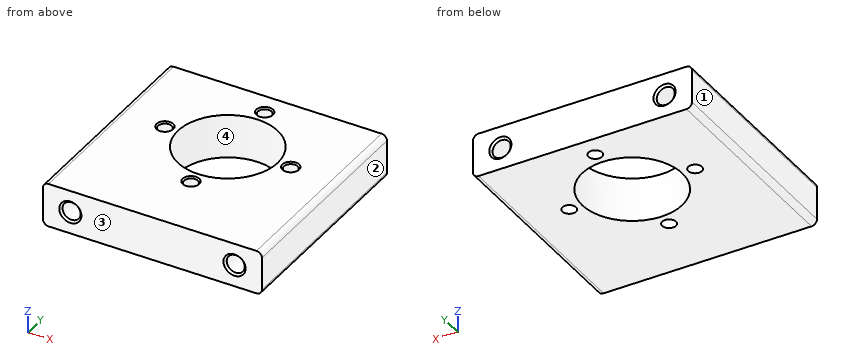
from build123d import *

# Parameters (mm, degrees)
SKETCH_1_W                   = 40
SKETCH_1_H                   = 8
EXTRUDE_1_DEPTH              = 39
HOLE_WIZARD_M4_1_D           = 3.3
HOLE_WIZARD_M4_1_DEPTH       = 9.108579979
HOLE_WIZARD_M4_1_CSINK_D     = 4.05
HOLE_WIZARD_M4_1_CSINK_ANGLE = 90
HOLE_WIZARD_M4_1_TIP         = 0.991420021
SKETCH_5_R                   = 9.125
CUT_EXTRUDE_1_DEPTH          = 39
HOLE_WIZARD_M4_2_D           = 3.3
HOLE_WIZARD_M4_2_DEPTH       = 9.108579979
HOLE_WIZARD_M4_2_CSINK_D     = 4.05
HOLE_WIZARD_M4_2_CSINK_ANGLE = 90
HOLE_WIZARD_M4_2_TIP         = 0.991420021
HOLE_WIZARD_M3_1_D           = 2.5
HOLE_WIZARD_M3_1_CSINK_D     = 3.05
HOLE_WIZARD_M3_1_CSINK_ANGLE = 90
FILLET_1_R                   = 1


with BuildPart() as part:
    # 草图1 → 凸台-拉伸1 (new body)
    with BuildSketch(Plane(origin=(0, 0, 0), x_dir=(1, 0, 0), z_dir=(0, 1, 0))):
        Rectangle(SKETCH_1_W, SKETCH_1_H)
    extrude(amount=EXTRUDE_1_DEPTH)

    # M4 螺纹孔1
    with Locations(Plane(origin=(0, 39, 0), x_dir=(1, 0, 0), z_dir=(0, 1, 0))):
        with Locations((-15, 0), (15, 0)):
            CounterSinkHole(HOLE_WIZARD_M4_1_D / 2, HOLE_WIZARD_M4_1_CSINK_D / 2, depth=HOLE_WIZARD_M4_1_DEPTH, counter_sink_angle=HOLE_WIZARD_M4_1_CSINK_ANGLE)
            with Locations((0, 0, -(HOLE_WIZARD_M4_1_DEPTH + HOLE_WIZARD_M4_1_TIP / 2))):  # 118° drill point
                Cone(0, HOLE_WIZARD_M4_1_D / 2, HOLE_WIZARD_M4_1_TIP, mode=Mode.SUBTRACT)

    # 草图5 → 切除-拉伸1 (cut)
    with BuildSketch(Plane.XY.offset(4)):
        with Locations((0, 23.5)):
            Circle(SKETCH_5_R)
    extrude(amount=-CUT_EXTRUDE_1_DEPTH, mode=Mode.SUBTRACT)

    # M4 螺纹孔2
    with Locations(Plane(origin=(0, 0, 0), x_dir=(-1, 0, 0), z_dir=(0, -1, 0))):
        with Locations((15, 0), (-15, 0)):
            CounterSinkHole(HOLE_WIZARD_M4_2_D / 2, HOLE_WIZARD_M4_2_CSINK_D / 2, depth=HOLE_WIZARD_M4_2_DEPTH, counter_sink_angle=HOLE_WIZARD_M4_2_CSINK_ANGLE)
            with Locations((0, 0, -(HOLE_WIZARD_M4_2_DEPTH + HOLE_WIZARD_M4_2_TIP / 2))):  # 118° drill point
                Cone(0, HOLE_WIZARD_M4_2_D / 2, HOLE_WIZARD_M4_2_TIP, mode=Mode.SUBTRACT)

    # M3 螺纹孔1 (through all)
    with Locations(Plane.XY.offset(4)):
        with Locations((0, 35), (-11.5, 23.5), (11.5, 23.5), (0, 12)):
            CounterSinkHole(HOLE_WIZARD_M3_1_D / 2, HOLE_WIZARD_M3_1_CSINK_D / 2, counter_sink_angle=HOLE_WIZARD_M3_1_CSINK_ANGLE)

    # 圆角1
    fillet_1_edges = [part.edges().sort_by_distance(p)[0] for p in [
        (20, 19.5, 4),
        (-20, 19.5, 4),
        (-20, 19.5, -4),
        (20, 19.5, -4),
    ]]
    fillet(fillet_1_edges, radius=FILLET_1_R)


solid = part.part
Model file for the job. Use its own axes, mm. Face numbers are marked on the shaded views. Give positions to 0.01 mm unless a question says otherwise; leave off trailing zeros. Order: outer loops, then holes, each group sorted by start corner. A loop starts at its lowest first (then second) coordinate and runs counter-clockwise, first axis right, second up. Notation, with made-up numbers: M -34.5,47.5 L -16.5,47.5 A35 cw -16.5,85.5 Z; hole C 73,-33 d11. An arc over 180 degrees is marked long. Write item = value, one per line.
Q1. Drill centre lines: line 1 (Z direction, x = -15, y = 36); line 2 (Y direction, x = 0, z = 1.25) (3 decimals); line 3 (Y direction, x = 11.5, z = -0.5). Where is each one in solid material? Low to high. Write a range as [from, to].
Derived:
line_1 = [-4, -1.65], [1.65, 4]
line_2 = [0, 10.75], [13.25, 14.375], [32.625, 33.75], [36.25, 39]
line_3 = [0, 22.25], [24.75, 39]
Q2. Cut at B-B, the plane x = -11.5. List the corners of the cut face in (y, z) (3 decimals).
Derived:
outline = M 0,-4 L 22.25,-4 L 22.25,3.725 L 21.975,4 L 0,4 Z; M 24.75,-4 L 39,-4 L 39,4 L 25.025,4 L 24.75,3.725 Z
Q3. Two-plate mould, pull along X, no slides. Class the marked faces 1, 2, 3 and 4: pulls with the +X half, pulls with the -X half, needs draft (parallel to the pull), parting line crosses it, or undercut.
Derived:
face_1 = pulls with the -X half
face_2 = pulls with the +X half
face_3 = needs draft
face_4 = undercut
Q4. Flat gauge pins, fed straight in: pin 1 (4 mm diameter, centred on x = -15, z = 0, fed in from -Y) (3 decimals); pin 2 (2 mm diameter, centred on x = 15, z = 0, fed in from +Y); pin 3 (2.5 mm diameter, centred on x = 15, z = 0, fed in from -Y). Where does each tip first touch, or does it go through?
Derived:
pin_1 = 0.025
pin_2 = 29.5
pin_3 = 9.35
Q5. Cut at C-C, the plane y = 12. List the corners of the cut face in (x, z) (3 decimals).
Derived:
outline = M -20,-3 A1 ccw -19,-4 L -1.25,-4 L -1.25,3.725 L -1.525,4 L -19,4 A1 ccw -20,3 Z; M 1.25,-4 L 19,-4 A1 ccw 20,-3 L 20,3 A1 ccw 19,4 L 1.525,4 L 1.25,3.725 Z
Q6. Cut at D-D, the plane z = -2.5. List the corners of the cut face in (x, y) (3 decimals).
Derived:
outline = M -20,0 L 20,0 L 20,39 L -20,39 Z; hole C -11.5,23.5 d2.5; hole C 0,23.5 d18.25; hole C 0,12 d2.5; hole C 0,35 d2.5; hole C 11.5,23.5 d2.5
Q7. Cut at A-A, the plane y = 35. List the corners of the cut face in (x, z) (3 decimals).
Derived:
outline = M -20,-3 A1 ccw -19,-4 L -1.25,-4 L -1.25,3.725 L -1.525,4 L -19,4 A1 ccw -20,3 Z; M 1.25,-4 L 19,-4 A1 ccw 20,-3 L 20,3 A1 ccw 19,4 L 1.525,4 L 1.25,3.725 Z; hole C -15,0 d3.3; hole C 15,0 d3.3
